```python
from build123d import *

# Parameters (mm, degrees)
SKETCH2_W                                           = 150
SKETCH2_H                                           = 30
BOSS_EXTRUDE1_DEPTH                                 = 30
SKETCH3_R                                           = 13.75
CUT_EXTRUDE1_DEPTH                                  = 23
LPATTERN1_COUNT                                     = 5
LPATTERN1_PITCH                                     = 30
CBORE_FOR_M4_HEX_SOCKET_HEAD_CAP_SCREW1_D           = 4.5
CBORE_FOR_M4_HEX_SOCKET_HEAD_CAP_SCREW1_CBORE_D     = 8
CBORE_FOR_M4_HEX_SOCKET_HEAD_CAP_SCREW1_CBORE_DEPTH = 4.4
LPATTERN2_COUNT                                     = 2
LPATTERN2_PITCH                                     = 120
SKETCH7_W                                           = 181.12901383
SKETCH7_H                                           = 4
CUT_EXTRUDE3_DEPTH                                  = 23
SKETCH8_W                                           = 4
SKETCH8_H                                           = 50
CUT_EXTRUDE4_DEPTH                                  = 23
SKIZZE1_R                                           = 16
SKIZZE1_R_2                                         = 15
SCHNITT_LINEAR_AUSTRAGEN1_DEPTH                     = 80.868642157
LPATTERN3_COUNT                                     = 5
LPATTERN3_PITCH                                     = 30
CBORE_FOR_M6_HEX_SOCKET_HEAD_CAP_SCREW1_D           = 6.6
CBORE_FOR_M6_HEX_SOCKET_HEAD_CAP_SCREW1_CBORE_D     = 11
CBORE_FOR_M6_HEX_SOCKET_HEAD_CAP_SCREW1_CBORE_DEPTH = 4.4
LPATTERN4_COUNT                                     = 2
LPATTERN4_PITCH                                     = 75
SKIZZE2_W                                           = 30
SKIZZE2_H                                           = 30
SCHNITT_LINEAR_AUSTRAGEN2_DEPTH                     = 30
SKIZZE3_W                                           = 30
SKIZZE3_H                                           = 30
SCHNITT_LINEAR_AUSTRAGEN3_DEPTH                     = 30


with BuildPart() as part:
    # Sketch2 → Boss-Extrude1 (new body)
    with BuildSketch(Plane(origin=(0, 0, 0), x_dir=(1, 0, 0), z_dir=(0, 1, 0))):
        Rectangle(SKETCH2_W, SKETCH2_H)
    extrude(amount=BOSS_EXTRUDE1_DEPTH)

    # Sketch3 → Cut-Extrude1 (cut)
    with BuildSketch(Plane(origin=(0, 30, 0), x_dir=(1, 0, 0), z_dir=(0, 1, 0))):
        with Locations(Location((-60, 0, 0), (0, 0, 270))):
            Circle(SKETCH3_R)
    cut_extrude1 = extrude(amount=-CUT_EXTRUDE1_DEPTH, mode=Mode.SUBTRACT)

    # LPattern1: Cut-Extrude1 ×5
    with Locations(*[(i * LPATTERN1_PITCH, 0, 0) for i in range(1, LPATTERN1_COUNT)]):
        add(cut_extrude1, mode=Mode.SUBTRACT)

    # CBORE for M4 Hex Socket Head Cap Screw1 (through all)
    with Locations(Plane(origin=(0, 7, 0), x_dir=(-1, 0, 0), z_dir=(0, 1, 0))):
        with Locations((60, 0)):
            cbore_for_m4_hex_socket_head_cap_screw1 = CounterBoreHole(CBORE_FOR_M4_HEX_SOCKET_HEAD_CAP_SCREW1_D / 2, CBORE_FOR_M4_HEX_SOCKET_HEAD_CAP_SCREW1_CBORE_D / 2, CBORE_FOR_M4_HEX_SOCKET_HEAD_CAP_SCREW1_CBORE_DEPTH)

    # LPattern2: CBORE for M4 Hex Socket Head Cap Screw1 ×2
    with Locations(*[(i * LPATTERN2_PITCH, 0, 0) for i in range(1, LPATTERN2_COUNT)]):
        add(cbore_for_m4_hex_socket_head_cap_screw1, mode=Mode.SUBTRACT)

    # Sketch7 → Cut-Extrude3 (cut)
    with BuildSketch(Plane(origin=(0, 30, 0), x_dir=(1, 0, 0), z_dir=(0, 1, 0))):
        Rectangle(SKETCH7_W, SKETCH7_H)
    extrude(amount=-CUT_EXTRUDE3_DEPTH, mode=Mode.SUBTRACT)

    # Sketch8 → Cut-Extrude4 (cut)
    with BuildSketch(Plane(origin=(0, 30, 0), x_dir=(-1, 0, 0), z_dir=(0, 1, 0))):
        with Locations((60, -1.298701607)):
            Rectangle(SKETCH8_W, SKETCH8_H)
    cut_extrude4 = extrude(amount=-CUT_EXTRUDE4_DEPTH, mode=Mode.SUBTRACT)

    # Skizze1 → Schnitt-Linear austragen1 (cut, through all)
    with BuildSketch(Plane(origin=(0, 7, 0), x_dir=(-1, 0, 0), z_dir=(0, 1, 0))):
        with Locations((60, 0)):
            Circle(SKIZZE1_R)
        with Locations((60, 0)):
            Circle(SKIZZE1_R_2, mode=Mode.SUBTRACT)
    schnitt_linear_austragen1 = extrude(amount=SCHNITT_LINEAR_AUSTRAGEN1_DEPTH, mode=Mode.SUBTRACT)

    # LPattern3: Cut-Extrude4, Schnitt-Linear austragen1 ×5
    with Locations(*[(i * LPATTERN3_PITCH, 0, 0) for i in range(1, LPATTERN3_COUNT)]):
        add(cut_extrude4, mode=Mode.SUBTRACT)
        add(schnitt_linear_austragen1, mode=Mode.SUBTRACT)

    # CBORE for M6 Hex Socket Head Cap Screw1 (through all)
    with Locations(Plane(origin=(0, 7, 0), x_dir=(-1, 0, 0), z_dir=(0, 1, 0))):
        with Locations((37.5, 0)):
            cbore_for_m6_hex_socket_head_cap_screw1 = CounterBoreHole(CBORE_FOR_M6_HEX_SOCKET_HEAD_CAP_SCREW1_D / 2, CBORE_FOR_M6_HEX_SOCKET_HEAD_CAP_SCREW1_CBORE_D / 2, CBORE_FOR_M6_HEX_SOCKET_HEAD_CAP_SCREW1_CBORE_DEPTH)

    # LPattern4: CBORE for M6 Hex Socket Head Cap Screw1 ×2
    with Locations(*[(i * LPATTERN4_PITCH, 0, 0) for i in range(1, LPATTERN4_COUNT)]):
        add(cbore_for_m6_hex_socket_head_cap_screw1, mode=Mode.SUBTRACT)

    # Skizze2 → Schnitt-Linear austragen2 (cut)
    with BuildSketch(Plane.ZY.offset(75)):
        with Locations((0, 15)):
            Rectangle(SKIZZE2_W, SKIZZE2_H)
    extrude(amount=-SCHNITT_LINEAR_AUSTRAGEN2_DEPTH, mode=Mode.SUBTRACT)

    # Skizze3 → Schnitt-Linear austragen3 (cut)
    with BuildSketch(Plane(origin=(75, 0, 0), x_dir=(0, 0, -1), z_dir=(1, 0, 0))):
        with Locations((0, 15)):
            Rectangle(SKIZZE3_W, SKIZZE3_H)
    extrude(amount=-SCHNITT_LINEAR_AUSTRAGEN3_DEPTH, mode=Mode.SUBTRACT)


solid = part.part
```
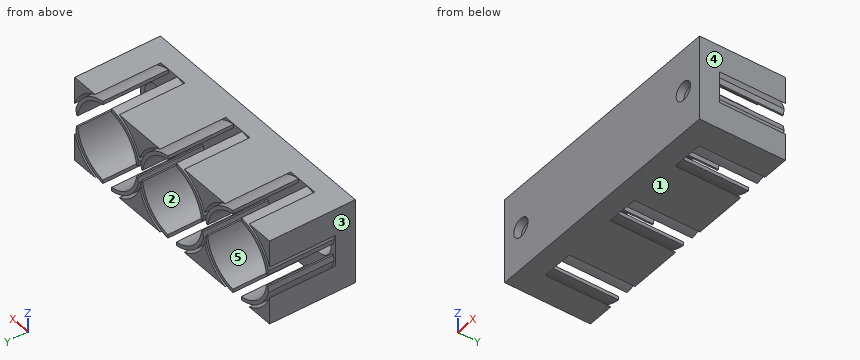
Check sheet for the modelled part. Datum: model origin and axes. Units: mm. Face numbers are marked on the shaded views. A direction names the side the tool comes from. Coordinates: 2 decimals unless noted, no trailing zeros. Order: outer loops, then holes, each group sorted by start corner. A loop starts at its lowest first (then second) coordinate and runs counter-clockwise, first axis right, second up. Notation, with made-up numbers: M 59.25,34 L 113.25,34 A13 cw 113.25,54 Z; hole C 59.5,-9 d1. An arc over 180 degrees is marked long. Write each question's results on one line, items separated by ' | '. Start each with the question number.
1. Cross-section at C-C on y = 27.5. State how many separate pieces and enclosed holes the cut face has, and give its area (3 significant figures).
2. Mould release check, pull along Z, two halves, no side actions. Record for the marked faces 1, 2 and 3: +Z half, -Z half, draft (parallel to the pull), parting line (faces both ways), or undercut.
3. Material ranges on probe 1 along Z at (x, y) = (37.5, 1.4); probe 2 along Z at (x, y) = (-37.5, 3.95); probe 3 along X at (y, z) = (4.75, -1.5), recorded low to high.
4. Cross-section at A-A on z = 0. Record the cut outline in (x, y), and give its area (3 significant figures).
5. Access from +Z, -Z, +X, -X, +Y, -Y to the whole of each face (thin tool, end or side, straight path). Record for the marked faces 4 and 5.
6. Go/stop test with flat-tipped pins: P1, Ø10, axis at x = 28, z = 4.5, coming from the -Y side; P2, Ø1, axis at y = 23, z = -3, coming from the +X side. Record where each tip stops, or that it passes through.
7. Cross-section at D-D on x = -10. Record the cut outline in (y, z), and give its area (3 significant figures).
8. Cross-section at B-B on x = -37.5. Record the cut outline in (y, z).
Checks:
1) separate pieces: 20 | enclosed holes: 0 | area: 646 mm²
2) face 1: -Z half | face 2: undercut | face 3: draft
3) probe 1: z = -15 to -3.3, 3.3 to 15 | probe 2: z = -15 to -5.5, 5.5 to 15 | probe 3: x = -45 to -42.79, -32.21 to 32.21, 42.79 to 45
4) outline: M -45,0 L -40.8,0 L -40.8,2.6 L -43,2.6 L -43,7 L -45,7 Z; M -34.2,0 L 34.2,0 L 34.2,2.6 L 32,2.6 L 32,7 L -32,7 L -32,2.6 L -34.2,2.6 Z; M 40.8,0 L 45,0 L 45,7 L 43,7 L 43,2.6 L 40.8,2.6 Z | area: 499 mm²
5) face 4: +Z, -Z, +X, +Y, -Y | face 5: +Y
6) P1: stops at y = 0 | P2: stops at x = 44.39
7) outline: M 0,-15 L 30,-15 L 30,-12.49 L 7,-12.49 L 7,-11.18 L 30,-11.18 L 30,-9.44 L 7,-9.44 L 7,9.44 L 30,9.44 L 30,11.18 L 7,11.18 L 7,12.49 L 30,12.49 L 30,15 L 0,15 Z | area: 406 mm²
8) outline: M 0,-15 L 30,-15 L 30,-14.13 L 7,-14.13 L 7,-12.99 L 30,-12.99 L 30,-11.52 L 7,-11.52 L 7,-5.5 L 2.6,-5.5 L 2.6,-3.3 L 0,-3.3 Z; M 0,3.3 L 2.6,3.3 L 2.6,5.5 L 7,5.5 L 7,11.52 L 30,11.52 L 30,12.99 L 7,12.99 L 7,14.13 L 30,14.13 L 30,15 L 0,15 Z
